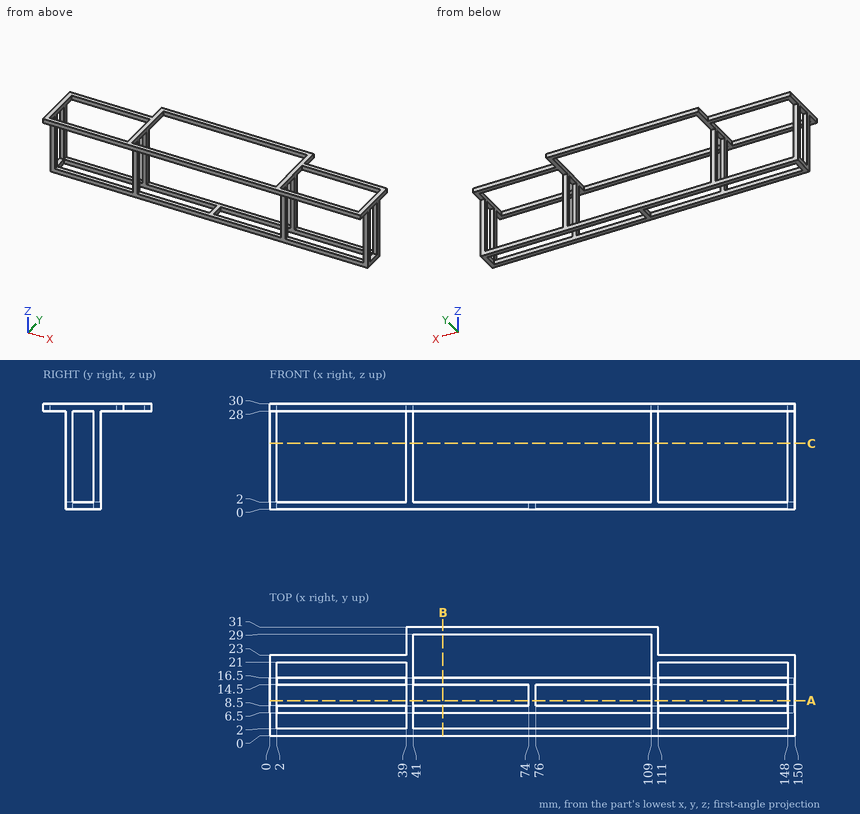
Geometry: see drawing. Coordinates: mm, zero at the bounding-box minimum. Give positions to 0.01 mm unless a question says otherwise; leave off trailing zeros. Loops run counter-clockwise (first coordinate to the right, second up) from the corner with the lowest first, then second, coordinate; pieces in that order, holes last. Notation, with made-up numbers: (39.25, 62) - (59.25, 62) arc R15 ccw to (59.25, 91) - close; hole circle Ø11 at (33, -11). An arc over 180 degrees is marked (long way). One line per question, with ' | ' between items. Start each with the question number.
(1) Section query B-B on x = 49.5. Return loops of the section in (y, z).
(2) Section query C-C on z = 18.75. Count the separate pieces of the cut face and the enclosed holes in it, then the cut area to 3 significant figures.
(3) Contact query for flat-ended pins moving along their axis: pin 1 (1.6 mm diameter, centred on x = 149.5, z = 9, fed in from +Y); pin 2 (2 mm diameter, centred on x = 77.5, z = 28.5, fed in from -Y); pin 3 (1 mm diameter, centred on x = 123.5, z = 28.5, fed in from +Y); pin 4 (2 mm diameter, centred on x = 1.5, z = 12, fed in from -Y). Output: stop coordinate, or through.
(4) Section query A-A on y = 10. Return loops of the section in (x, z), then the cut area to 3 significant figures.
(5) Ray query, line 1 (X direction, y = 7, z = 16.75); line 2 (Y direction, x = 66, z = 28.75); line 3 (Y direction, x = 142.5, z = 1.5). Return the intervals inside material, ascending. Write a range as from..to.
The answers:
1) outline: (0, 28) - (2, 28) - (2, 30) - (0, 30) - close; (6.5, 0) - (8.5, 0) - (8.5, 2) - (6.5, 2) - close; (14.5, 0) - (16.5, 0) - (16.5, 2) - (14.5, 2) - close; (29, 28) - (31, 28) - (31, 30) - (29, 30) - close
2) separate pieces: 8 | enclosed holes: 0 | area: 32.0 mm2
3) pin 1: y = 16.5 | pin 2: y = 0 | pin 3: y = 23 | pin 4: y = 6.5
4) outline: (0, 0) - (2, 0) - (2, 2) - (0, 2) - close; (0, 28) - (2, 28) - (2, 30) - (0, 30) - close; (39, 28) - (41, 28) - (41, 30) - (39, 30) - close; (74, 0) - (76, 0) - (76, 2) - (74, 2) - close; (109, 28) - (111, 28) - (111, 30) - (109, 30) - close; (148, 0) - (150, 0) - (150, 2) - (148, 2) - close; (148, 28) - (150, 28) - (150, 30) - (148, 30) - close | area: 28.0 mm2
5) line 1: 0..2, 39..41, 109..111, 148..150 | line 2: 0..2, 29..31 | line 3: 6.5..8.5, 14.5..16.5
